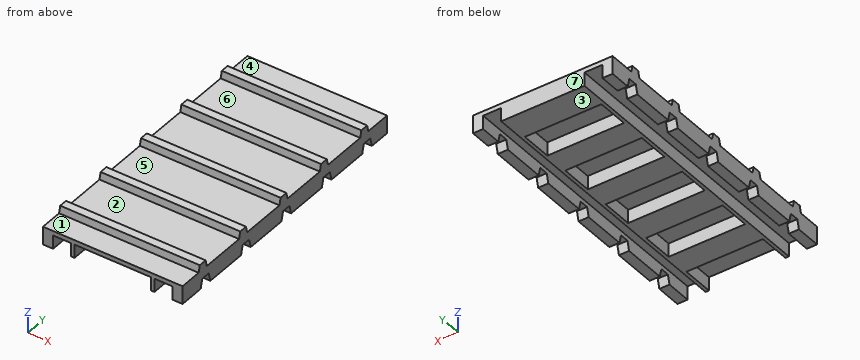
from build123d import *

# Parameters (mm, degrees)
SKETCH2_W                  = 34
SKETCH2_H                  = 13.32
BOSS_EXTRUDE1_DEPTH        = 4
SKETCH3_W                  = 17
SKETCH3_H                  = 7
CUT_EXTRUDE1_DEPTH         = 3
SKETCH4_W                  = 4
SKETCH4_H                  = 13.32
CUT_EXTRUDE3_DEPTH         = 3
CUT_EXTRUDE4_DEPTH         = 4
CUT_EXTRUDE5_DEPTH         = 4
BOSS_EXTRUDE2_DEPTH        = 34
SKETCH9_W                  = 1.5
SKETCH9_H                  = 13.32
CUT_EXTRUDE6_DEPTH         = 10
CRVPATTERN11_START         = -8.5
CRVPATTERN11_OUTLINE_W     = 0.77
CRVPATTERN11_OUTLINE_H     = 3
CRVPATTERN11_DEPTH         = 17
CRVPATTERN11_START_2       = -9.25
CRVPATTERN11_2_DEPTH       = 18.5
CRVPATTERN11_START_3       = -15.5
CRVPATTERN11_3_DEPTH       = 31
CRVPATTERN11_START_4       = 13.25
CRVPATTERN11_4_DEPTH       = 2.25
CRVPATTERN11_5_DEPTH       = 2.25
CRVPATTERN11_6_OUTLINE_W   = 7
CRVPATTERN11_6_OUTLINE_H   = 3
CRVPATTERN11_6_OUTLINE_W_2 = 6.23
CRVPATTERN11_6_DEPTH       = 0.75
CRVPATTERN11_START_5       = 8.5
CRVPATTERN11_7_OUTLINE_W   = 7
CRVPATTERN11_7_OUTLINE_H   = 3
CRVPATTERN11_7_OUTLINE_W_2 = 6.23
CRVPATTERN11_7_DEPTH       = 0.75


with BuildPart() as part:
    # Sketch2 → Boss-Extrude1 (new body)
    with BuildSketch(Plane.XY):
        with Locations((0, 6.66)):
            Rectangle(SKETCH2_W, SKETCH2_H)
    extrude(amount=BOSS_EXTRUDE1_DEPTH)

    # Sketch3 → Cut-Extrude1 (cut)
    with BuildSketch(Plane(origin=(0, 0, 0), x_dir=(-1, 0, 0), z_dir=(0, 0, -1))):
        with Locations((0, 3.5)):
            Rectangle(SKETCH3_W, SKETCH3_H)
    extrude(amount=-CUT_EXTRUDE1_DEPTH, mode=Mode.SUBTRACT)

    # Sketch4 → Cut-Extrude3 (cut)
    with BuildSketch(Plane(origin=(0, 0, 0), x_dir=(-1, 0, 0), z_dir=(0, 0, -1))):
        with Locations((-11.25, 6.66)):
            Rectangle(SKETCH4_W, SKETCH4_H)
        with Locations((11.25, 6.66)):
            Rectangle(SKETCH4_W, SKETCH4_H)
    extrude(amount=-CUT_EXTRUDE3_DEPTH, mode=Mode.SUBTRACT)

    # Sketch6 → Cut-Extrude4 (cut)
    with BuildSketch(Plane(origin=(17, 0, 0), x_dir=(0, 0, -1), z_dir=(1, 0, 0))):
        Polygon((0, 8.62), (0, 5.62), (-2, 6.12), (-2, 8.12), align=None)
    extrude(amount=-CUT_EXTRUDE4_DEPTH, mode=Mode.SUBTRACT)

    # Sketch7 → Cut-Extrude5 (cut)
    with BuildSketch(Plane.ZY.offset(17)):
        Polygon((0, 5.616283946), (0, 8.62), (2, 8.117101335), (2, 6.119182611), align=None)
    extrude(amount=-CUT_EXTRUDE5_DEPTH, mode=Mode.SUBTRACT)

    # Sketch8 → Boss-Extrude2 (add)
    with BuildSketch(Plane.ZY.offset(17)):
        Polygon((4, 5), (4, 7.5), (5.5, 7.15), (5.5, 5.35), align=None)
    extrude(amount=-BOSS_EXTRUDE2_DEPTH)

    # Sketch9 → Cut-Extrude6 (cut)
    with BuildSketch(Plane(origin=(0, 0, 0), x_dir=(-1, 0, 0), z_dir=(0, 0, -1))):
        with Locations((-16.25, 6.66)):
            Rectangle(SKETCH9_W, SKETCH9_H)
        with Locations((16.25, 6.66)):
            Rectangle(SKETCH9_W, SKETCH9_H)
    extrude(amount=-CUT_EXTRUDE6_DEPTH, mode=Mode.SUBTRACT)

    # CrvPattern11: read off the stored shape, not the designer's step
    # CrvPattern11 outline → CrvPattern11 (cut)
    with BuildSketch(Plane.YZ.offset(CRVPATTERN11_START)):
        with Locations((12.935, 1.5)):
            Rectangle(CRVPATTERN11_OUTLINE_W, CRVPATTERN11_OUTLINE_H)
    extrude(amount=CRVPATTERN11_DEPTH, mode=Mode.SUBTRACT)

    # CrvPattern11 2 outline → CrvPattern11 2 (add)
    with BuildSketch(Plane.YZ.offset(CRVPATTERN11_START_2)):
        Polygon((55.2, 4), (45.15, 4), (44.8, 5.5), (43, 5.5), (42.65, 4), (32.6, 4), (32.25, 5.5), (30.45, 5.5), (30.1, 4), (20.05, 4), (19.7, 5.5), (17.9, 5.5), (17.55, 4), (13.32, 4), (13.32, 3), (19.55, 3), (19.55, 0), (25.1, 0), (25.1, 3), (32.1, 3), (32.1, 0), (37.65, 0), (37.65, 3), (44.65, 3), (44.65, 0), (50.2, 0), (50.2, 3), (57.2, 3), (57.2, 0), (63.52, 0), (63.52, 4), (57.7, 4), (57.35, 5.5), (55.55, 5.5), align=None)
    extrude(amount=CRVPATTERN11_2_DEPTH)

    # CrvPattern11 3 outline → CrvPattern11 3 (add)
    with BuildSketch(Plane.YZ.offset(CRVPATTERN11_START_3)):
        Polygon((55.2, 4), (45.15, 4), (44.8, 5.5), (43, 5.5), (42.65, 4), (32.6, 4), (32.25, 5.5), (30.45, 5.5), (30.1, 4), (20.05, 4), (19.7, 5.5), (17.9, 5.5), (17.55, 4), (13.32, 4), (13.32, 3), (63.52, 3), (63.52, 4), (57.7, 4), (57.35, 5.5), (55.55, 5.5), align=None)
    extrude(amount=CRVPATTERN11_3_DEPTH)

    # CrvPattern11 4 outline → CrvPattern11 4 (add)
    with BuildSketch(Plane.YZ.offset(CRVPATTERN11_START_4)):
        Polygon((63.52, 0), (63.52, 3), (13.32, 3), (13.32, 0), (18.17, 0), (18.67, 2), (20.67, 2), (21.17, 0), (30.72, 0), (31.22, 2), (33.22, 2), (33.72, 0), (43.27, 0), (43.77, 2), (45.77, 2), (46.27, 0), (55.82, 0), (56.32, 2), (58.32, 2), (58.82, 0), align=None)
    extrude(amount=CRVPATTERN11_4_DEPTH)

    # CrvPattern11 5 outline → CrvPattern11 5 (add)
    with BuildSketch(Plane.YZ.offset(CRVPATTERN11_START_3)):
        Polygon((63.52, 0), (63.52, 3), (13.32, 3), (13.32, 0), (18.166283946, 0), (18.669182611, 2), (20.667101335, 2), (21.17, 0), (30.716283946, 0), (31.219182611, 2), (33.217101335, 2), (33.72, 0), (43.266283946, 0), (43.769182611, 2), (45.767101335, 2), (46.27, 0), (55.816283946, 0), (56.319182611, 2), (58.317101335, 2), (58.82, 0), align=None)
    extrude(amount=CRVPATTERN11_5_DEPTH)

    # CrvPattern11 6 outline → CrvPattern11 6 (add)
    with BuildSketch(Plane.YZ.offset(CRVPATTERN11_START_2)):
        with Locations((53.7, 1.5)):
            Rectangle(CRVPATTERN11_6_OUTLINE_W, CRVPATTERN11_6_OUTLINE_H)
        with Locations((41.15, 1.5)):
            Rectangle(CRVPATTERN11_6_OUTLINE_W, CRVPATTERN11_6_OUTLINE_H)
        with Locations((28.6, 1.5)):
            Rectangle(CRVPATTERN11_6_OUTLINE_W, CRVPATTERN11_6_OUTLINE_H)
        with Locations((16.435, 1.5)):
            Rectangle(CRVPATTERN11_6_OUTLINE_W_2, CRVPATTERN11_6_OUTLINE_H)
    extrude(amount=CRVPATTERN11_6_DEPTH)

    # CrvPattern11 7 outline → CrvPattern11 7 (add)
    with BuildSketch(Plane.YZ.offset(CRVPATTERN11_START_5)):
        with Locations((53.7, 1.5)):
            Rectangle(CRVPATTERN11_7_OUTLINE_W, CRVPATTERN11_7_OUTLINE_H)
        with Locations((41.15, 1.5)):
            Rectangle(CRVPATTERN11_7_OUTLINE_W, CRVPATTERN11_7_OUTLINE_H)
        with Locations((28.6, 1.5)):
            Rectangle(CRVPATTERN11_7_OUTLINE_W, CRVPATTERN11_7_OUTLINE_H)
        with Locations((16.435, 1.5)):
            Rectangle(CRVPATTERN11_7_OUTLINE_W_2, CRVPATTERN11_7_OUTLINE_H)
    extrude(amount=CRVPATTERN11_7_DEPTH)


solid = part.part
Input: part model. Units: mm. Frame: model coordinates. Face numbers are marked on the shaded views. A direction names the side the tool comes from. Coordinates: 2 decimals unless noted, no trailing zeros. Loops run counter-clockwise (first coordinate to the right, second up) from the corner with the lowest first, then second, coordinate; pieces in that order, holes last. Notation, with made-up numbers: (54, 4) -> (59, 4) arc R32 ccw to (59, 31) -> close; hole circle Ø1 at (21.5, 85.25). An arc over 180 degrees is marked (long way). One line per item, written item: value.
(1) Set-up query: the marked faces 1, 2 and 3. Return all of +Z, -Z, +X, -X, +Y, -Y with unobstructed straight access to the full face (end or side cutting, diameter ignored); none if empty.
Answer below:
face 1: +Z, +X, -X, -Y
face 2: +Z, +X, -X
face 3: -Z, +X, -X, +Y, -Y
(2) Cut plane B-B (z = 0.95). Give the number of separate pieces and of enclosed holes in the cut face, then the cut area to 3 significant figures.
Answer below:
separate pieces: 13
enclosed holes: 4
area: 809 mm2
(3) Ray query, line 1 along Y through (x, z) = (2, 2); line 2 along X through (y, z) = (23, 1); line 3 along Z through (x, y) = (-13.5, 13.5). Return the intervals inside material, ascending.
Answer below:
line 1: y = 7 to 12.55, 19.55 to 25.1, 32.1 to 37.65, 44.65 to 50.2, 57.2 to 63.52
line 2: x = -15.5 to -13.25, -9.25 to 9.25, 13.25 to 15.5
line 3: z = 0 to 4
(4) Cut plane C-C (y = 22). Output: boundary loops of the cut face in (x, z).
Answer below:
outline: (-15.5, 0) -> (-13.25, 0) -> (-13.25, 3) -> (-9.25, 3) -> (-9.25, 0) -> (9.25, 0) -> (9.25, 3) -> (13.25, 3) -> (13.25, 0) -> (15.5, 0) -> (15.5, 4) -> (-15.5, 4) -> close
(5) Pin query (flat end, axial travel): pin 1 Ø3 at (x, y) = (-0.5, 61) entering from +Z; pin 2 Ø5.5 at (x, y) = (-0.5, 2.5) entering from -Z; pin 3 Ø1 at (x, y) = (14, 20) entering from -Z. Return the tip coordinate at first contact, or that it passes through.
Answer below:
pin 1: stops at z = 4
pin 2: stops at z = 3
pin 3: stops at z = 2
(6) Cut plane A-A (y = 29). Output: boundary loops of the cut face in (x, z), then the cut area to 3 significant figures.
Answer below:
outline: (-15.5, 0) -> (-13.25, 0) -> (-13.25, 3) -> (-9.25, 3) -> (-9.25, 0) -> (-8.5, 0) -> (-8.5, 3) -> (8.5, 3) -> (8.5, 0) -> (9.25, 0) -> (9.25, 3) -> (13.25, 3) -> (13.25, 0) -> (15.5, 0) -> (15.5, 4) -> (-15.5, 4) -> close
area: 49.0 mm2
(7) Draft query along Y for the marked faces 4, 5, 6 and 7. Return one class per face: pulls with the +Y half, pulls with the -Y half, needs draft (parallel to the pull), parting line crosses it, or undercut.
Answer below:
face 4: needs draft
face 5: undercut
face 6: undercut
face 7: pulls with the +Y half
